Input: part model. Units: mm. Frame: model coordinates. A direction names the side the tool comes from. Round coordinates to 2 decimals unless told otherwise and drop trailing zeros. Order: outer loops, then holes, each group sorted by start corner. A loop starts at its lowest first (then second) coordinate and runs counter-clockwise, first axis right, second up. Notation, with made-up numbers: (-16.75, 75) -> (-2.75, 75) arc R24 cw to (-2.75, 110) -> close; hole circle Ø6 at (-7, 6.25). An arc over 180 degrees is marked (long way). Use a Markdown table: item, result.
from build123d import *

# Parameters (mm, degrees)
SKETCH_1_W          = 54
SKETCH_1_H          = 54
EXTRUDE_1_DEPTH     = 27
SKETCH_2_W          = 54
SKETCH_2_H          = 54
SKETCH_2_W_2        = 18
SKETCH_2_H_2        = 18
CUT_EXTRUDE_1_DEPTH = 54
SKETCH_3_W          = 18
SKETCH_3_H          = 36
CUT_EXTRUDE_2_DEPTH = 34.674916481
FILLET_1_R          = 1
SCALE_1_SCALE       = 2.083333333
SKETCH_5_W          = 33.333333334
SKETCH_5_H          = 33.333333334
CUT_EXTRUDE_3_DEPTH = 2
SKETCH_6_R          = 3
CUT_EXTRUDE_4_DEPTH = 6


with BuildPart() as part:
    # 草图1 → 凸台-拉伸1 (new, symmetric)
    with BuildSketch(Plane.XY):
        Rectangle(SKETCH_1_W, SKETCH_1_H)
    extrude(amount=EXTRUDE_1_DEPTH, both=True)

    # 草图2 → 切除-拉伸1 (cut)
    with BuildSketch(Plane(origin=(0, 27, 0), x_dir=(1, 0, 0), z_dir=(0, 1, 0))):
        Rectangle(SKETCH_2_W, SKETCH_2_H)
        Rectangle(SKETCH_2_W_2, SKETCH_2_H_2, mode=Mode.SUBTRACT)
    extrude(amount=-CUT_EXTRUDE_1_DEPTH, mode=Mode.SUBTRACT)

    # 草图3 → 切除-拉伸2 (cut, through all)
    with BuildSketch(Plane.XY.offset(9)):
        with Locations((0, -9)):
            Rectangle(SKETCH_3_W, SKETCH_3_H)
    extrude(amount=-CUT_EXTRUDE_2_DEPTH, mode=Mode.SUBTRACT)

    # 草图4 → 切除-旋转1 (revolve, cut)
    with BuildSketch(Plane.XY):
        with BuildLine():
            Line((0, 25), (0, -25))
            ThreePointArc((0, -25), (-25, 0), (0, 25))
        make_face()
    revolve(axis=Axis((0, 25, 0), (0, -1, 0)), mode=Mode.SUBTRACT)

    # 圆角1
    fillet_1_edges = [part.edges().sort_by_distance(p)[0] for p in [
        (9, 27, 0),
        (0, 27, 9),
        (-9, 27, 0),
        (0, 27, -9),
    ]]
    fillet(fillet_1_edges, radius=FILLET_1_R)


with BuildPart() as part_1:
    # 缩放比例1: scaled about (0, 0, 0)
    add(part.part.scale(SCALE_1_SCALE))

    # 草图5 → 切除-拉伸3 (cut)
    with BuildSketch(Plane(origin=(0, 56.25, 0), x_dir=(1, 0, 0), z_dir=(0, 1, 0))):
        Rectangle(SKETCH_5_W, SKETCH_5_H)
    extrude(amount=-CUT_EXTRUDE_3_DEPTH, mode=Mode.SUBTRACT)

    # 草图6 → 切除-拉伸4 (cut)
    with BuildSketch(Plane(origin=(0, 54.25, 0), x_dir=(1, 0, 0), z_dir=(0, 1, 0))):
        with Locations(Location((0, 0, 0), (0, 0, 270))):
            Circle(SKETCH_6_R)
    extrude(amount=-CUT_EXTRUDE_4_DEPTH, mode=Mode.SUBTRACT)


solid = part_1.part
1) Line query: L1, parallel to X at y = 52.75, z = 0; L2, parallel to X at y = 54.75, z = -10. Output: solid intervals per line, ascending. Write a range as [from, to].
Results found:
| item | result |
|---|---|
| L1 | x = [-18.75, -3], [3, 18.75] |
| L2 | x = [-18.67, -16.67], [16.67, 18.67] |
2) Set-up query: faces 1 (the cylindrical face through (0.9, 53.14, 2.86)), 2 (the flat face through (0, 55, -16.667)). Return all of +Z, -Z, +X, -X, +Y, -Y with unobstructed straight access to the full face (end or side cutting, diameter ignored); none if empty.
Results found:
| item | result |
|---|---|
| face 1 | +Y, -Y |
| face 2 | +Y |
3) Pin query (flat end, axial travel): pin 1 Ø7 at (x, z) = (0, 0) entering from -Y; pin 2 Ø6 at (x, z) = (-6, -12.5) entering from -Y; pin 3 Ø1 at (y, z) = (55, 0.5) entering from +X. Return the tip coordinate at first contact, or that it passes through.
Results found:
| item | result |
|---|---|
| pin 1 | stops at y = 51.97 |
| pin 2 | stops at y = 49.28 |
| pin 3 | stops at x = 18.72 |
4) Cut plane A-A on y = 55.25. Return loops of the section in (x, z).
Results found:
| item | result |
|---|---|
| outline | (-18.45, -18.45) -> (18.45, -18.45) -> (18.45, 18.45) -> (-18.45, 18.45) -> close; hole (-16.67, -16.67) -> (16.67, -16.67) -> (16.67, 16.67) -> (-16.67, 16.67) -> close |
5) Cut plane B-B on z = -1. Return loops of the section in (x, y).
Results found:
| item | result |
|---|---|
| outline | (-18.75, 48.58) arc R52.07 cw to (-2.83, 52) -> (-2.83, 54.25) -> (-16.67, 54.25) -> (-16.67, 56.25) arc R2.08 ccw to (-18.75, 54.17) -> close; (2.83, 52) arc R52.07 cw to (18.75, 48.58) -> (18.75, 54.17) arc R2.08 ccw to (16.67, 56.25) -> (16.67, 54.25) -> (2.83, 54.25) -> close |
6) Cut plane C-C on x = 0. Return loops of the section in (y, z), and give its area (3 significant figures).
Results found:
| item | result |
|---|---|
| outline | (48.59, -18.75) -> (54.17, -18.75) arc R2.08 ccw to (56.25, -16.67) -> (54.25, -16.67) -> (54.25, -3) -> (52, -3) arc R52.08 cw to start; (48.59, 18.75) arc R52.08 cw to (52, 3) -> (54.25, 3) -> (54.25, 16.67) -> (56.25, 16.67) arc R2.08 ccw to (54.17, 18.75) -> close |
| area | 118 mm² |
7) Cut plane D-D on x = -10.5. Return loops of the section in (y, z).
Results found:
| item | result |
|---|---|
| outline | (47.44, -18.75) -> (54.17, -18.75) arc R2.08 ccw to (56.25, -16.67) -> (54.25, -16.67) -> (54.25, 16.67) -> (56.25, 16.67) arc R2.08 ccw to (54.17, 18.75) -> (47.44, 18.75) arc R51.01 cw to start |
8) Pull-direction query (X, two-part tool) for faces 3 (the flat face through (16.667, 55, 0)), 4 (the flat face through (18.75, 51, 0)), 5 (the flat face through (-18.75, 51, 0)), 6 (the flat face through (0, 51, -18.75)); classes: +X half, -X half, draft (parallel to the pull), parting line (faces both ways), or undercut.
Results found:
| item | result |
|---|---|
| face 3 | undercut |
| face 4 | +X half |
| face 5 | -X half |
| face 6 | draft |
